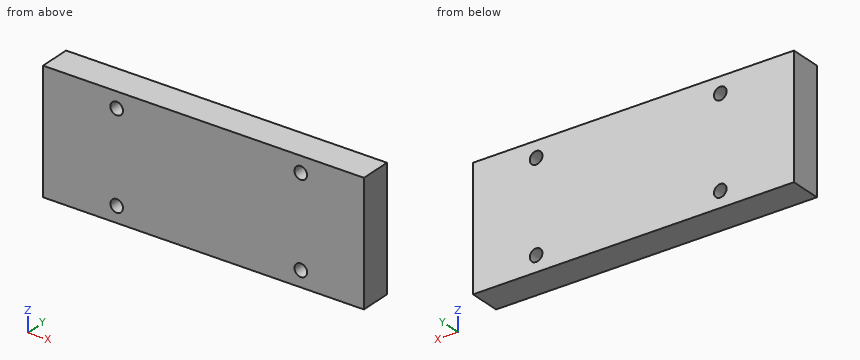
```python
from build123d import *

# Parameters (mm, degrees)
CYLINDER001_R     = 1.2
CYLINDER001_DEPTH = 10
CYLINDER002_R     = 1.2
CYLINDER002_DEPTH = 10
CYLINDER003_R     = 1.2
CYLINDER003_DEPTH = 10
CYLINDER_R        = 1.2
CYLINDER_DEPTH    = 10
BOX002_W          = 61
BOX002_H          = 6
BOX002_DEPTH      = 23


with BuildPart() as m2s001:
    # Cylinder001 → Cylinder001 (new body)
    with BuildSketch(Plane(origin=(14, 0, 20), x_dir=(1, 0, 0), z_dir=(0, -1, 0))):
        Circle(CYLINDER001_R)
    extrude(amount=CYLINDER001_DEPTH)


with BuildPart() as m2s002:
    # Cylinder002 → Cylinder002 (new body)
    with BuildSketch(Plane(origin=(49, 0, 20), x_dir=(1, 0, 0), z_dir=(0, -1, 0))):
        Circle(CYLINDER002_R)
    extrude(amount=CYLINDER002_DEPTH)


with BuildPart() as m2s003:
    # Cylinder003 → Cylinder003 (new body)
    with BuildSketch(Plane(origin=(49, 0, 3), x_dir=(1, 0, 0), z_dir=(0, -1, 0))):
        Circle(CYLINDER003_R)
    extrude(amount=CYLINDER003_DEPTH)


with BuildPart() as obj1:
    # Cylinder → Cylinder (new body)
    with BuildSketch(Plane(origin=(14, 0, 3), x_dir=(1, 0, 0), z_dir=(0, -1, 0))):
        Circle(CYLINDER_R)
    extrude(amount=CYLINDER_DEPTH)

    # Fusion: union m2s001, m2s002, m2s003
    add(m2s001.part)
    add(m2s002.part)
    add(m2s003.part)


with BuildPart() as obj1_1:
    # Fusion placement: moved
    add(obj1.part.moved(Location((0, 6, 0))))


with BuildPart() as e5mini:
    # Box002 → Box002 (new body)
    with BuildSketch(Plane.XY):
        with Locations((30.5, 3)):
            Rectangle(BOX002_W, BOX002_H)
    extrude(amount=BOX002_DEPTH)

    # Cut: cut obj1
    add(obj1_1.part, mode=Mode.SUBTRACT)


with BuildPart() as e5mini_1:
    # Cut placement: moved
    add(e5mini.part.moved(Location((30, 5.7, 15))))


solid = e5mini_1.part
```
Work out the finished part from the listing and answer in its coordinate system (mm). Give positions to 0.01 mm unless a question says otherwise; leave off trailing zeros. Order: outer loops, then holes, each group sorted by start corner. A loop starts at its lowest first (then second) coordinate and runs counter-clockwise, first axis right, second up. Notation, with made-up numbers: (-12, -19.75) -> (37, -19.75) arc R16 cw to (37, -9.75) -> close; hole circle Ø3 at (85, 50.5). An arc over 180 degrees is marked (long way). Answer as CSV lines item,"result". Start each with the question number.
(1) Each of these flat-tipped pins is pushed along its axis until it touches: pin 1 Ø3 at (x, z) = (44, 35) entering from +Y; pin 2 Ø1.9 at (x, z) = (79, 35) entering from -Y. Where does it stop, or does it pass through?
(2) Section A-A, the plane z = 35 is taken. Write down the section's boundary in (x, y).
(3) Section B-B, the plane x = 79 is taken. Write down the section's boundary in (y, z), plus the area to 3 significant figures.
(4) Consider line 1 along X through (y, z) = (9.3, 35); line 2 along Z through (x, y) = (79, 7.45); line 3 along X through (y, z) = (6, 36). Determine where each line is inside the solid, lowest interval first.
Entries:
1,pin 1,"y = 11.7"
1,pin 2,"through"
2,outline,"(30, 5.7) -> (42.8, 5.7) -> (42.8, 11.7) -> (30, 11.7) -> close; (45.2, 5.7) -> (77.8, 5.7) -> (77.8, 11.7) -> (45.2, 11.7) -> close; (80.2, 5.7) -> (91, 5.7) -> (91, 11.7) -> (80.2, 11.7) -> close"
3,outline,"(5.7, 15) -> (11.7, 15) -> (11.7, 16.8) -> (5.7, 16.8) -> close; (5.7, 19.2) -> (11.7, 19.2) -> (11.7, 33.8) -> (5.7, 33.8) -> close; (5.7, 36.2) -> (11.7, 36.2) -> (11.7, 38) -> (5.7, 38) -> close"
3,area,"109 mm²"
4,line 1,"30 to 42.8, 45.2 to 77.8, 80.2 to 91"
4,line 2,"15 to 16.8, 19.2 to 33.8, 36.2 to 38"
4,line 3,"30 to 43.34, 44.66 to 78.34, 79.66 to 91"
